Build history of the part. All positions in model axes, mm. Face numbers are marked on the shaded views. Give positions to 0.01 mm unless a question says otherwise; leave off trailing zeros. Order: outer loops, then holes, each group sorted by start corner. A loop starts at its lowest first (then second) coordinate and runs counter-clockwise, first axis right, second up. Notation, with made-up numbers: (88.25, 69) - (113.25, 69) arc R31 cw to (113.25, 93) - close; hole circle Ø8 at (15, 26). An arc over 180 degrees is marked (long way). Write each question's results on one line, items separated by ' | '. Start each with the question number.
Autodesk Inventor part; units mm, degrees
ref_plane "YZ Plane" through (0, 0, 0) normal (1, 0, 0) x (0, 1, 0)
ref_plane "XZ Plane" through (0, 0, 0) normal (0, 1, 0) x (-1, 0, 0)
ref_plane "XY Plane" through (0, 0, 0) normal (0, 0, 1) x (1, 0, 0)
sketch "Sketch1" plane through (0, 0, 0) normal (0, 1, 0) x (-1, 0, 0)
  line L0 (3, 9.5) -> (-3, 9.5)
  line L1 (-3, 9.5) -> (-3, -9.5)
  line L2 (-3, -9.5) -> (3, -9.5)
  line L3 (3, -9.5) -> (3, 9.5)
  line L4 (3, 9.5) -> (-3, -9.5) construction
  line L5 (-3, 9.5) -> (3, -9.5) construction
  circle A0 centre (0, 9.5) radius 3
  circle A1 centre (0, -9.5) radius 3
  line L6 (-3, -9.5) -> (-7, -9.5)
  line L7 (-7, -9.5) -> (-7, -5.5)
  line L8 (-7, -5.5) -> (-7, -3.5)
  line L9 (-7, -3.5) -> (-3, -3.5)
  line L10 (-7, -3.5) -> (-7, -6.5)
  circle A2 centre (-7, -6.5) radius 3
  line L11 (-3, -3.5) -> (-3, -9.5)
  point P0 (0, 0)
  dimension "d0" = 6
  dimension "d1" = 19
  dimension "d2" = 6
  dimension "d4" = 6
  dimension "d5" = 4
  dimension "d6" = 4
  dimension "d7" = 2
  dimension "d10" = 3
  dimension "d11" = 6
extrude "Extrusion1" add sketch "Sketch1" along normal blind 1.5 contours A0 L0 | L0 A0 | L3 A1 L1 A0 | A1 L2 | L2 A1 | A2 L7 L8 | L8 L7 A2
sketch "Sketch2" plane through (0, 1.5, 0) normal (0, 1, 0) x (1, 0, 0)
  line L0 (3, -9.5) -> (3, 9.5)
  arc A0 (3, 9.5) -> (-3, 9.5) centre (0, 9.5) ccw
  line L1 (-3, 9.5) -> (-3, -9.5)
  arc A1 (-3, -9.5) -> (3, -9.5) centre (0, -9.5) ccw
  circle A2 centre (0, 9.5) radius 1.5
  circle A3 centre (0, -9.5) radius 1.5
  line L2 (3, 9.5) -> (7, 9.5)
  line L3 (7, 9.5) -> (7, 3.5)
  line L4 (7, 3.5) -> (3, 3.5)
  line L5 (3, 3.5) -> (3, 9.5)
  point P0 (0, 0)
  dimension "d14" = 3
  dimension "d15" = 3
  dimension "d16" = 4
  dimension "d17" = 6
extrude "Extrusion2" cut sketch "Sketch2" against normal blind 1.5 contours L0 L2 L3 L4 | A2 | A3
sketch "Sketch3" plane through (0, 1.5, 0) normal (0, 1, 0) x (1, 0, 0)
  line L0 (3, -9.5) -> (3, 9.5)
  arc A0 (3, 9.5) -> (-3, 9.5) centre (0, 9.5) ccw
  line L1 (-3, 9.5) -> (-3, -9.5)
  line L2 (3, 9.5) -> (7, 9.5)
  line L3 (7, 9.5) -> (7, 3.5)
  line L4 (7, 3.5) -> (3, 3.5)
  line L5 (3, 3.5) -> (3, 9.5)
  point P0 (0, 0)
  dimension "d20" = 4
  dimension "d21" = 6
  dimension "d22" = 4
extrude "Extrusion3" add sketch "Sketch3" against normal blind 1.5
sketch "Sketch4" plane through (0, 1.5, 0) normal (0, 1, 0) x (1, 0, 0)
  arc A0 (7, 3.5) -> (7, 9.5) centre (7, 6.5) ccw
  circle A1 centre (7, 6.5) radius 1.5
  point P0 (0, 0)
  dimension "d25" = 3
extrude "Extrusion4" cut sketch "Sketch4" against normal blind 1.5
sketch "Sketch5" plane through (0, 0, 0) normal (0, -1, 0) x (1, 0, 0)
  circle A0 centre (7, -6.5) radius 1.5
  circle A1 centre (0, 9.5) radius 1.5
  circle A2 centre (0, -9.5) radius 1.5
  arc A3 (7, -9.5) -> (7, -3.5) centre (7, -6.5) ccw
  arc A4 (3, 9.5) -> (-3, 9.5) centre (0, 9.5) ccw
  arc A5 (-3, -9.5) -> (3, -9.5) centre (0, -9.5) ccw
  circle A6 centre (0, 9.5) radius 0.1
  circle A7 centre (0, -9.5) radius 0.1
  circle A8 centre (7, -6.5) radius 0.1
  point P0 (0, 0)
  dimension "d28" = 0.2
  dimension "d29" = 0.2
  dimension "d30" = 0.2
extrude "Extrusion5" add sketch "Sketch5" against normal blind 1.5
properties part number "tahlo3_sablona_19"
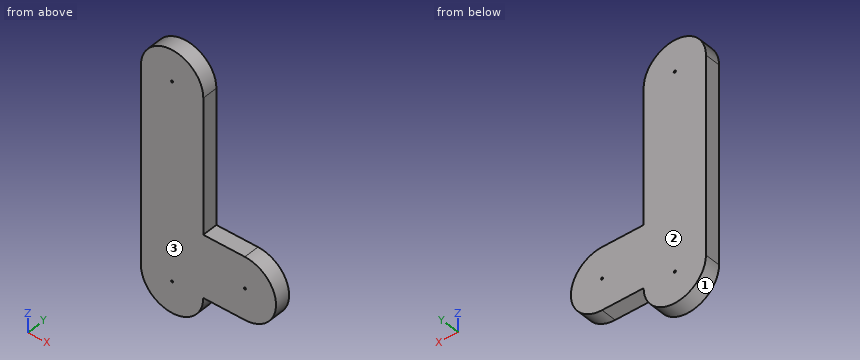
Item 1: Cut at A-A, the plane y = 0.85. List the corners of the cut face in (x, z), then the cut area to 3 significant figures.
Item 2: Cut at C-C, the plane x = 6. List the corners of the cut face in (y, z).
Item 3: Probe line 1 along Z through (x, y) = (0, 0.85); line 2 along X through (y, z) = (0.6, 9.5); line 3 along Z through (x, y) = (7, 1.25). List the from-to ranges inside material, lowest first. Write a range as from..to.
Item 4: Cut at B-B, the plane z = 4. List the corners of the cut face in (x, y).
Item 5: Flat gauge pin, fed straight in: pin 1 Ø0.8 at (x, y) = (4.5, 0.5) entering from +Z. Where does the tip first touch, or does it go through?
Item 6: Two-plate mould, pull along Y, no slides. Class the marked faces 1, 2 and 3: +Y half, -Y half, draft (parallel to the pull), parting line (faces both ways), or undercut.
Values found:
1) outline: (-3, -9.5) arc R3 ccw to (3, -9.5) - (7, -9.5) arc R3 ccw to (7, -3.5) - (3, -3.5) - (3, 9.5) arc R3 ccw to (-3, 9.5) - close; hole circle Ø0.2 at (0, -9.5); hole circle Ø0.2 at (0, 9.5); hole circle Ø0.2 at (7, -6.5) | area: 180 mm2
2) outline: (0, -9.5) - (1.5, -9.5) - (1.5, -3.5) - (0, -3.5) - close
3) line 1: z = -12.5..-9.6, -9.4..9.4, 9.6..12.5 | line 2: x = -3..-0.1, 0.1..3 | line 3: z = -9.5..-6.6, -6.4..-3.5
4) outline: (-3, 0) - (3, 0) - (3, 1.5) - (-3, 1.5) - close
5) pin 1: stops at z = -3.5
6) face 1: draft | face 2: +Y half | face 3: -Y half
